```python
from build123d import *

# Parameters (mm, degrees)
F0_R     = 4.601152
F0_R_2   = 1
F0_R_3   = 1.5
F1_DEPTH = 7.6
F2_DEPTH = 7.25
F3_DEPTH = 7.55
F4_DEPTH = 7.55
F5_DEPTH = 7.55
F6_DEPTH = 7.25
F0_R_4   = 4.190001
F7_DEPTH = 7


with BuildPart() as f1:
    # F0 (on Front) → F1 (new body)
    with BuildSketch(Plane.XZ):
        with BuildLine():
            Line((-18.595, -60.475), (18.595, -60.475))
            ThreePointArc((18.595, -60.475), (25.135738, -57.765738), (27.845, -51.225))
            Line((27.845, -51.225), (27.845, 51.225))
            ThreePointArc((27.845, 51.225), (25.135738, 57.765738), (18.595, 60.475))
            Line((18.595, 60.475), (-18.595, 60.475))
            ThreePointArc((-18.595, 60.475), (-25.135738, 57.765738), (-27.845, 51.225))
            Line((-27.845, 51.225), (-27.845, -51.225))
            ThreePointArc((-27.845, -51.225), (-25.135738, -57.765738), (-18.595, -60.475))
        make_face()
        with Locations((0, -52.765)):
            Circle(F0_R, mode=Mode.SUBTRACT)
        with Locations((-8.015, 52.259863)):
            Circle(F0_R_2, mode=Mode.SUBTRACT)
        with BuildLine():
            ThreePointArc((25.85, -44.15), (25.557107, -44.857107), (24.85, -45.15))
            Line((24.85, -45.15), (-24.85, -45.15))
            ThreePointArc((-24.85, -45.15), (-25.557107, -44.857107), (-25.85, -44.15))
            Line((-25.85, -44.15), (-25.85, 44.15))
            ThreePointArc((-25.85, 44.15), (-25.557107, 44.857107), (-24.85, 45.15))
            Line((-24.85, 45.15), (24.85, 45.15))
            ThreePointArc((24.85, 45.15), (25.557107, 44.857107), (25.85, 44.15))
            Line((25.85, 44.15), (25.85, -44.15))
        make_face(mode=Mode.SUBTRACT)
        with BuildLine():
            Line((-4.405, 53.409863), (4.405, 53.409863))
            ThreePointArc((4.405, 53.409863), (5.112107, 53.11697), (5.405, 52.409863))
            Line((5.405, 52.409863), (5.405, 52.109863))
            ThreePointArc((5.405, 52.109863), (5.112107, 51.402756), (4.405, 51.109863))
            Line((4.405, 51.109863), (-4.405, 51.109863))
            ThreePointArc((-4.405, 51.109863), (-5.112107, 51.402756), (-5.405, 52.109863))
            Line((-5.405, 52.109863), (-5.405, 52.409863))
            ThreePointArc((-5.405, 52.409863), (-5.112107, 53.11697), (-4.405, 53.409863))
        make_face(mode=Mode.SUBTRACT)
        with Locations((0, 55.845)):
            Circle(F0_R_3, mode=Mode.SUBTRACT)
    extrude(amount=F1_DEPTH)

    # F0 (on Front) → F2 (join)
    with BuildSketch(Plane.XZ):
        with BuildLine():
            Line((-18.535, -61.915), (18.535, -61.915))
            ThreePointArc((18.535, -61.915), (26.136398, -58.766398), (29.285, -51.165))
            Line((29.285, -51.165), (29.285, 51.165))
            ThreePointArc((29.285, 51.165), (26.136398, 58.766398), (18.535, 61.915))
            Line((18.535, 61.915), (-18.535, 61.915))
            ThreePointArc((-18.535, 61.915), (-26.136398, 58.766398), (-29.285, 51.165))
            Line((-29.285, 51.165), (-29.285, -51.165))
            ThreePointArc((-29.285, -51.165), (-26.136398, -58.766398), (-18.535, -61.915))
        make_face()
        with BuildLine():
            ThreePointArc((27.845, -51.225), (25.135738, -57.765738), (18.595, -60.475))
            Line((18.595, -60.475), (-18.595, -60.475))
            ThreePointArc((-18.595, -60.475), (-25.135738, -57.765738), (-27.845, -51.225))
            Line((-27.845, -51.225), (-27.845, 51.225))
            ThreePointArc((-27.845, 51.225), (-25.135738, 57.765738), (-18.595, 60.475))
            Line((-18.595, 60.475), (18.595, 60.475))
            ThreePointArc((18.595, 60.475), (25.135738, 57.765738), (27.845, 51.225))
            Line((27.845, 51.225), (27.845, -51.225))
        make_face(mode=Mode.SUBTRACT)
    extrude(amount=F2_DEPTH)

    # F0 (on Front) → F3 (join)
    with BuildSketch(Plane.XZ):
        with BuildLine():
            Line((-24.85, -45.15), (24.85, -45.15))
            ThreePointArc((24.85, -45.15), (25.557107, -44.857107), (25.85, -44.15))
            Line((25.85, -44.15), (25.85, 44.15))
            ThreePointArc((25.85, 44.15), (25.557107, 44.857107), (24.85, 45.15))
            Line((24.85, 45.15), (-24.85, 45.15))
            ThreePointArc((-24.85, 45.15), (-25.557107, 44.857107), (-25.85, 44.15))
            Line((-25.85, 44.15), (-25.85, -44.15))
            ThreePointArc((-25.85, -44.15), (-25.557107, -44.857107), (-24.85, -45.15))
        make_face()
    extrude(amount=F3_DEPTH)

    # F0 (on Front) → F4 (join)
    with BuildSketch(Plane.XZ):
        with Locations((0, 55.845)):
            Circle(F0_R_3)
    extrude(amount=F4_DEPTH)

    # F0 (on Front) → F5 (join)
    with BuildSketch(Plane.XZ):
        with Locations((-8.015, 52.259863)):
            Circle(F0_R_2)
    extrude(amount=F5_DEPTH)

    # F0 (on Front) → F6 (join)
    with BuildSketch(Plane.XZ):
        with BuildLine():
            ThreePointArc((5.405, 52.409863), (5.112107, 53.11697), (4.405, 53.409863))
            Line((4.405, 53.409863), (-4.405, 53.409863))
            ThreePointArc((-4.405, 53.409863), (-5.112107, 53.11697), (-5.405, 52.409863))
            Line((-5.405, 52.409863), (-5.405, 52.109863))
            ThreePointArc((-5.405, 52.109863), (-5.112107, 51.402756), (-4.405, 51.109863))
            Line((-4.405, 51.109863), (4.405, 51.109863))
            ThreePointArc((4.405, 51.109863), (5.112107, 51.402756), (5.405, 52.109863))
            Line((5.405, 52.109863), (5.405, 52.409863))
        make_face()
    extrude(amount=F6_DEPTH)


with BuildPart() as f7:
    # F0 (on Front) → F7 (new body)
    with BuildSketch(Plane.XZ):
        with Locations((0, -52.765)):
            Circle(F0_R_4)
    extrude(amount=F7_DEPTH)


solid = f1.part
```
Check sheet for the modelled part. Datum: model origin and axes. Units: mm. A direction names the side the tool comes from. Round coordinates to 2 decimals unless told otherwise and drop trailing zeros. Order: outer loops, then holes, each group sorted by start corner. A loop starts at its lowest first (then second) coordinate and runs counter-clockwise, first axis right, second up. Notation, with made-up numbers: (47, 51.5) -> (57, 51.5) arc R4 cw to (57, 57.5) -> close; hole circle Ø3 at (15, 57.5). An arc over 180 degrees is marked (long way). One line per item, written item: value. Start each with the question number.
Q1. Mould release check, pull along X, two halves, no side actions. Record for faces 1 (the face through (26.2, -3.6, 58.7)), 2 (the face through (0, -7.25, 52)): pulls with the +X half, pulls with the -X half, needs draft (parallel to the pull), parting line crosses it, or undercut.
Q2. Cross-section at A-A (x = 0). Record the boundary of the cut face in (y, z) (3 decimals), and give its area (3 significant figures).
Q3. Set-up check for faces 3 (the face through (-25.2, -7.4, -57.7)), 4 (the face through (25.1, -7.4, -57.8)), 5 (the face through (-25.1, -7.4, 57.8)): record each of +Z, -Z, +X, -X, +Y, -Y from which the full face is reachable in a straight line by a thin tool's end or side.
Q4. Cross-section at B-B (y = -4). Record the boundary of the cut face in (x, z) (3 decimals), and give its area (3 significant figures).
Q5. Gauge pin test, flat ends, axial feed: pin 1 Ø8.5 at (x, z) = (0, -52.765) entering from -Y; pin 2 Ø1.5 at (x, z) = (-15, 12.5) entering from -Y; pin 3 Ø1.2 at (x, z) = (-1.5, 52.5) entering from -Y. Record the tip position at first contact, or that the pin passes through.
Q6. Thickness scan on line 1 (Y direction, x = -20.5, z = 35); line 2 (Z direction, x = -3.5, y = -4.25) (3 decimals); line 3 (X direction, y = -0.25, z = 53.5). Record the ranges inside material, lowest first.
Completed:
1. face 1: pulls with the +X half
1. face 2: undercut
2. outline: (-7.6, -60.475) -> (-7.25, -60.475) -> (-7.25, -61.915) -> (0, -61.915) -> (0, -57.366) -> (-7.6, -57.366) -> close; (-7.6, -48.164) -> (0, -48.164) -> (0, 61.915) -> (-7.25, 61.915) -> (-7.25, 60.475) -> (-7.6, 60.475) -> (-7.6, 57.345) -> (-7.55, 57.345) -> (-7.55, 54.345) -> (-7.6, 54.345) -> (-7.6, 53.41) -> (-7.25, 53.41) -> (-7.25, 51.11) -> (-7.6, 51.11) -> (-7.6, 45.15) -> (-7.55, 45.15) -> (-7.55, -45.15) -> (-7.6, -45.15) -> close
2. area: 865 mm²
3. face 3: -Z, -X, -Y
3. face 4: -Z, +X, -Y
3. face 5: +Z, -X, -Y
4. outline: (-29.285, -51.165) arc R10.75 ccw to (-18.535, -61.915) -> (18.535, -61.915) arc R10.75 ccw to (29.285, -51.165) -> (29.285, 51.165) arc R10.75 ccw to (18.535, 61.915) -> (-18.535, 61.915) arc R10.75 ccw to (-29.285, 51.165) -> close; hole circle Ø9.202 at (0, -52.765)
4. area: 7,090 mm²
5. pin 1: passes through
5. pin 2: stops at y = -7.55
5. pin 3: stops at y = -7.25
6. line 1: y = -7.55 to 0
6. line 2: z = -61.915 to -55.752, -49.778 to 61.915
6. line 3: x = -29.03 to 29.03
